```python
from build123d import *

# Parameters (mm, degrees)
SKETCH1_R           = 25.4
SKETCH1_R_2         = 19.05
BOSS_EXTRUDE1_DEPTH = 21.59
FILLET1_R           = 2.54
SKETCH2_W           = 2.54
SKETCH2_H           = 17.90600611
BOSS_EXTRUDE2_DEPTH = 5.08


with BuildPart() as part:
    # Sketch1 → Boss-Extrude1 (new body, symmetric)
    with BuildSketch(Plane(origin=(0, 0, 0), x_dir=(0, 0, -1), z_dir=(1, 0, 0))):
        Circle(SKETCH1_R)
        Circle(SKETCH1_R_2, mode=Mode.SUBTRACT)
    extrude(amount=BOSS_EXTRUDE1_DEPTH, both=True)

    # Fillet1
    fillet1_edges = [part.edges().sort_by_distance(p)[0] for p in [
        (-21.59, 0, 25.4),
        (21.59, 0, 25.4),
    ]]
    fillet(fillet1_edges, radius=FILLET1_R)

    # Sketch2 → Boss-Extrude2 (add, symmetric)
    with BuildSketch(Plane(origin=(0, 0, 0), x_dir=(0, 0, -1), z_dir=(1, 0, 0))):
        with Locations((0, 13.871691905)):
            Rectangle(SKETCH2_W, SKETCH2_H)
        Polygon((1.863681184, 4.72579014), (3.918584349, 3.232815599), (14.443470668, 17.719078843), (12.388567502, 19.212053384), align=None)
        Polygon((4.285499499, 2.72780022), (5.070402665, 0.312116669), (22.100026457, 5.845376858), (21.315123291, 8.26106041), align=None)
        Polygon((5.070402665, -0.312116669), (4.285499499, -2.72780022), (21.315123291, -8.26106041), (22.100026457, -5.845376858), align=None)
        Polygon((3.918584349, -3.232815599), (1.863681184, -4.72579014), (12.388567502, -19.212053384), (14.443470668, -17.719078843), align=None)
        with Locations((0, -13.871691905)):
            Rectangle(SKETCH2_W, SKETCH2_H)
        Polygon((-1.863681184, -4.72579014), (-3.918584349, -3.232815599), (-14.443470668, -17.719078843), (-12.388567502, -19.212053384), align=None)
        Polygon((-4.285499499, -2.72780022), (-5.070402665, -0.312116669), (-22.100026457, -5.845376858), (-21.315123291, -8.26106041), align=None)
        Polygon((-5.070402665, 0.312116669), (-4.285499499, 2.72780022), (-21.315123291, 8.26106041), (-22.100026457, 5.845376858), align=None)
        Polygon((-3.918584349, 3.232815599), (-1.863681184, 4.72579014), (-12.388567502, 19.212053384), (-14.443470668, 17.719078843), align=None)
    extrude(amount=BOSS_EXTRUDE2_DEPTH, both=True)

    # Sketch3 → Revolve1 (revolve)
    with BuildSketch(Plane(origin=(0, 0, 0), x_dir=(0, 0, -1), z_dir=(1, 0, 0))):
        with BuildLine():
            Line((0, 8.255), (0, -8.255))
            ThreePointArc((0, -8.255), (8.255, 0), (0, 8.255))
        make_face()
    revolve(axis=Axis((0, 8.255, 0), (0, -1, 0)))


solid = part.part
```
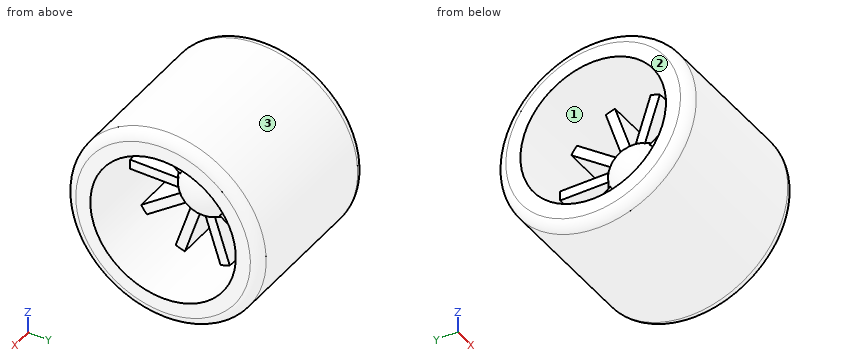
CAD build for the part. Positions are in the model's coordinates, mm. Face numbers are marked on the shaded views. Round coordinates to 2 decimals unless told otherwise and drop trailing zeros. Write each loop counter-clockwise with the first axis right and the second up, starting at its lowest first coordinate (ties: lowest second). Pieces come first, ordered by that corner, then holes. Notation, with made-up numbers: (77, -37.75) - (115, -37.75) arc R9 ccw to (115, -28.75) - close; hole circle Ø1 at (75.25, -19.75). An arc over 180 degrees is marked (long way). Write item = value, one per line. Start each with the question number.
Q1. Band-saw the part on C-C (z = 0). Give the cut face in (x, y) (3 decimals).
Q2. Drop flat-ended pins along their axis: pin 1 (5 mm diameter, centred on y = -5, z = 13.5, fed in from +X); pin 2 (2 mm diameter, centred on x = 3, y = -12.5, fed in from -Z); pin 3 (1 mm diameter, centred on y = -6, z = 12.5, fed in from +X); pin 4 (1.9 mm diameter, centred on y = -4, z = -15, fed in from -X). Give the stop position or say it passes through.
Q3. Probe L1, parallel to Y at x = 11, z = 0; L2, parallel to Y at x = 7.5, z = 0; L3, parallel to Y at x = 3, z = 12. List the from-to ranges inside material, lowest first. Write a range as from..to.
Q4. Mould opens along Z. For the marked faces 1, 2 and 3 say: pulls with the +Z half, pulls with the -Z half, needs draft (parallel to the pull), parting line crosses it, or undercut.
Q5. Band-saw the part on D-D (x = 7). Give the cut face in (y, z).
Q6. Band-saw the part on A-A (y = 0). Give the cut face in (x, z) (3 decimals), then the cut area to 3 significant figures.
Q7. Band-saw the part on B-B (x = 17.5). Give the cut face in (y, z), then the cut area to 3 significant figures.
Answers below:
q1.outline = (-21.59, -22.86) arc R2.54 ccw to (-19.05, -25.4) - (19.05, -25.4) arc R2.54 ccw to (21.59, -22.86) - (21.59, -19.05) - (5.08, -19.05) - (5.08, -6.507) arc R8.255 ccw to (5.08, 6.507) - (5.08, 19.05) - (21.59, 19.05) - (21.59, 22.86) arc R2.54 ccw to (19.05, 25.4) - (-19.05, 25.4) arc R2.54 ccw to (-21.59, 22.86) - (-21.59, 19.05) - (-5.08, 19.05) - (-5.08, 6.507) arc R8.255 ccw to (-5.08, -6.507) - (-5.08, -19.05) - (-21.59, -19.05) - close
q2.pin_1 = 5.08
q2.pin_2 = -22.65
q2.pin_3 = through
q2.pin_4 = -5.08
q3.L1 = -25.4..-19.05, 19.05..25.4
q3.L2 = -25.4..-19.05, -3.45..3.45, 19.05..25.4
q3.L3 = -22.39..-14.36, -5.23..-2.56, 2.56..5.23, 14.36..22.39
q4.face_1 = undercut
q4.face_2 = needs draft
q4.face_3 = parting line crosses it
q5.outline = circle Ø50.8 at (0, 0); circle Ø8.75 at (0, 0); hole circle Ø38.1 at (0, 0)
q6.outline = (-21.59, -22.86) arc R2.54 ccw to (-19.05, -25.4) - (19.05, -25.4) arc R2.54 ccw to (21.59, -22.86) - (21.59, -19.05) - (-21.59, -19.05) - close; (-21.59, 19.05) - (21.59, 19.05) - (21.59, 22.86) arc R2.54 ccw to (19.05, 25.4) - (-19.05, 25.4) arc R2.54 ccw to (-21.59, 22.86) - close; circle Ø16.51 at (0, 0)
q6.area = 757 mm2
q7.outline = circle Ø50.8 at (0, 0); hole circle Ø38.1 at (0, 0)
q7.area = 887 mm2
